Source: CAD feature listing. Evaluate the final solid. Frame: model axes, mm. Face numbers are marked on the shaded views. A direction names the side the tool comes from. Round coordinates to 2 decimals unless told otherwise and drop trailing zeros. Loops run counter-clockwise (first coordinate to the right, second up) from the corner with the lowest first, then second, coordinate; pieces in that order, holes last. Notation, with made-up numbers: M -18,19.25 L 8,19.25 A21 ccw 8,30.25 Z; hole C 62,-36.5 d8. An arc over 180 degrees is marked long. Write each question's results on one line, items separated by ' | '. Start each with the question number.
1. Section D-D on y = 3.25. Give the number of separate pieces and of enclosed holes in the cut face, and give its area (3 significant figures).
2. Section A-A on z = -15.5. Output: boundary loops of the cut face in (x, y), and give its area (3 significant figures).
3. Set-up query: the marked faces 1, 2 and 3. Return all of +Z, -Z, +X, -X, +Y, -Y with unobstructed straight access to the full face (end or side cutting, diameter ignored); none if empty.
4. Ray query, line 1 (X direction, y = 15.25, z = -12); line 2 (Z direction, x = -17.5, y = 5.75); line 3 (Z direction, x = -21, y = 0.5). Return the intervals inside material, ascending.
5. Draft query along Z for the marked faces 4, 5, 6 and 7. Return one class per face: released by +Z, released by -Z, zero draft, split by the parting line, or undercut.
6. Section B-B on x = 13.5. Output: boundary loops of the cut face in (y, z), and give its area (3 significant figures).
7. Section C-C on x = -4.5. Output: boundary loops of the cut face in (y, z), and give its area (3 significant figures).
8. Contact query for flat-ended pins moving along their axis: pin 1 Ø7.5 at (x, y) = (14, 14) entering from +Z; pin 2 Ø2 at (x, y) = (19, 1.5) entering from -Z; pin 3 Ø4 at (x, y) = (22, 13.5) entering from +Z. Output: stop coordinate, or through.
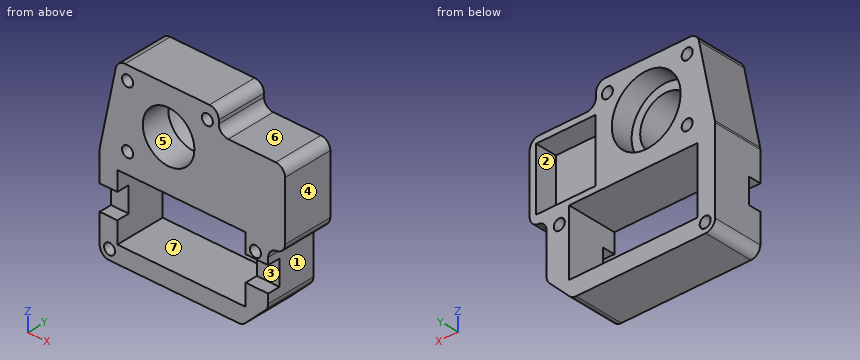
from build123d import *

# Parameters (mm, degrees)
ESBO_O1_R                = 8.25
ESBO_O1_R_2              = 1.759398981
ESBO_O1_W                = 41
ESBO_O1_H                = 21
RESSALTO_EXTRUS_O1_DEPTH = 16
ESBO_O2_R                = 11
ESBO_O2_W                = 19
ESBO_O2_H                = 20
CORTE_EXTRUS_O1_DEPTH    = 7
FILETE2_R                = 3
FILETE3_R                = 3
ESBO_O4_W                = 8
ESBO_O4_H                = 4
CORTE_EXTRUS_O2_DEPTH    = 60


with BuildPart() as part:
    # Esboço1 → Ressalto-extrusão1 (new body)
    with BuildSketch(Plane(origin=(0, 0, 0), x_dir=(1, 0, 0), z_dir=(0, 1, 0))):
        Polygon((-30, -1.447454982), (-30, 28.699395637), (15.649759457, 28.699395637), (23.854058099, 20.495096994), (23.854058099, 3.185553214), (29.26109124, 3.185553214), (29.26109124, -21.609914281), (8.073270411, -21.609914281), (8.073270411, -28.699395637), (-24.350240543, -28.699395637), align=None)
        with Locations((-7.979986437, -14.080173672)):
            Circle(ESBO_O1_R, mode=Mode.SUBTRACT)
        with Locations((-26.846540224, 25.498704653)):
            Circle(ESBO_O1_R_2, mode=Mode.SUBTRACT)
        with Locations((19.799323859, 6.233376584)):
            Circle(ESBO_O1_R_2, mode=Mode.SUBTRACT)
        with Locations((-21.074944534, -24.259345494)):
            Circle(ESBO_O1_R_2, mode=Mode.SUBTRACT)
        with Locations((4.428183177, -24.259345494)):
            Circle(ESBO_O1_R_2, mode=Mode.SUBTRACT)
        with Locations((-21.074944534, -4.342364945)):
            Circle(ESBO_O1_R_2, mode=Mode.SUBTRACT)
        with Locations((-3.850240543, 12.685553214)):
            Rectangle(ESBO_O1_W, ESBO_O1_H, mode=Mode.SUBTRACT)
    extrude(amount=RESSALTO_EXTRUS_O1_DEPTH)

    # Esboço2 → Corte-extrusão1 (cut)
    with BuildSketch(Plane(origin=(0, 16, 0), x_dir=(1, 0, 0), z_dir=(0, 1, 0))):
        with Locations((-7.979986437, -14.080173672)):
            Circle(ESBO_O2_R)
        with Locations((17.716848977, -9.668999278)):
            Rectangle(ESBO_O2_W, ESBO_O2_H)
    extrude(amount=-CORTE_EXTRUS_O1_DEPTH, mode=Mode.SUBTRACT)

    # Filete2
    filete2_edges = [part.edges().sort_by_distance(p)[0] for p in [
        (-30, 8, 1.447454982),
        (-30, 8, -28.699395637),
        (15.649759457, 8, -28.699395637),
        (23.854058099, 8, -20.495096994),
        (23.854058099, 8, -3.185553214),
        (8.073270411, 8, 28.699395637),
        (-24.350240543, 8, 28.699395637),
    ]]
    fillet(filete2_edges, radius=FILETE2_R)

    # Filete3
    filete3_edges = [part.edges().sort_by_distance(p)[0] for p in [
        (29.26109124, 8, -3.185553214),
        (8.073270411, 8, 21.609914281),
        (29.26109124, 8, 21.609914281),
    ]]
    fillet(filete3_edges, radius=FILETE3_R)

    # Esboço4 → Corte-extrusão2 (cut)
    with BuildSketch(Plane.ZY.offset(30)):
        with Locations((-12.370867745, 2)):
            Rectangle(ESBO_O4_W, ESBO_O4_H)
    extrude(amount=-CORTE_EXTRUS_O2_DEPTH, mode=Mode.SUBTRACT)


solid = part.part
Taken from the geometry:
1) separate pieces: 2 | enclosed holes: 6 | area: 1,770 mm^2
2) outline: M -30,4 L -24.35,4 L -24.35,16 L -30,16 Z; M 16.65,4 L 23.85,4 L 23.85,16 L 16.65,16 Z | area: 154 mm^2
3) face 1: -Z, +X, +Y, -Y | face 2: +Y | face 3: +X, -X, -Y
4) line 1: -30 to -24.35, 16.65 to 23.85 | line 2: -28.7 to -23.19, -2.19 to 28.7 | line 3: -28.7 to -23.19, -2.19 to 2.58, 6.1 to 22.5, 26.02 to 28.7
5) face 4: zero draft | face 5: undercut | face 6: released by +Z | face 7: undercut
6) outline: M 0,-28.7 L 16,-28.7 L 16,-23.19 L 0,-23.19 Z; M 0,-2.19 L 16,-2.19 L 16,-0.33 L 9,-0.33 L 9,19.67 L 16,19.67 L 16,21.61 L 0,21.61 Z | area: 329 mm^2
7) outline: M 0,-28.7 L 16,-28.7 L 16,-23.19 L 0,-23.19 Z; M 0,-2.19 L 16,-2.19 L 16,3.65 L 9,3.65 L 9,6.6 L 0,6.6 Z; M 0,21.56 L 9,21.56 L 9,24.52 L 16,24.52 L 16,28.7 L 0,28.7 Z | area: 302 mm^2
8) pin 1: z = 21.73 | pin 2: z = -26.35 | pin 3: z = 21.61
